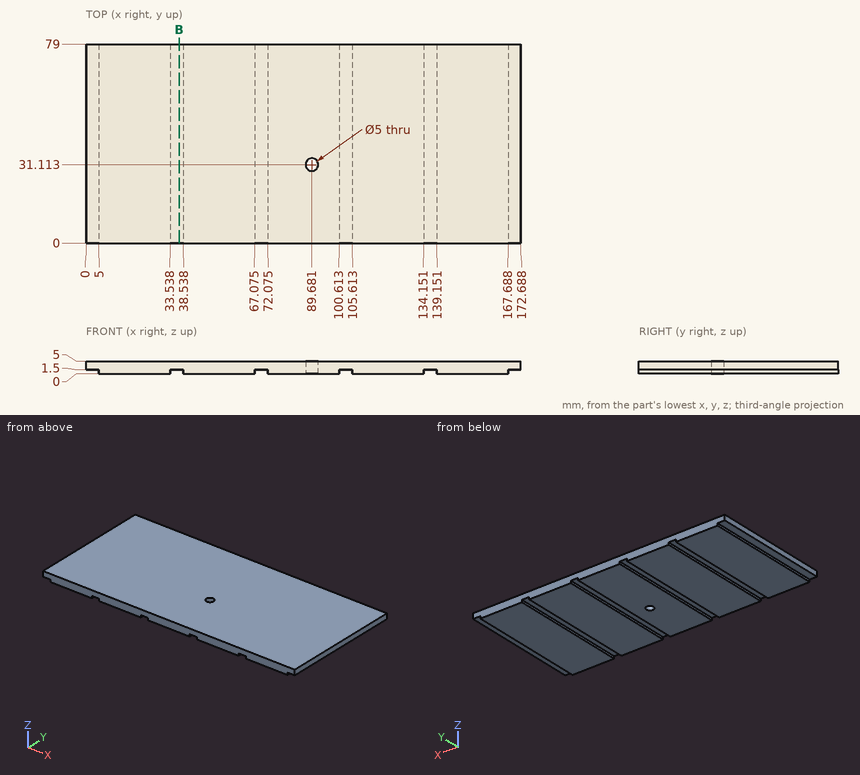
Can you work these out from the drawing? Everything is in mm from the part's minimum corner. Give positions to 0.01 mm unless a question says otherwise; leave off trailing zeros. Order: outer loops, then holes, each group sorted by start corner. A loop starts at its lowest first (then second) coordinate and runs counter-clockwise, first axis right, second up. Notation, with made-up numbers: M 38,65.25 L 72,65.25 A26 cw 72,91.25 Z; hole C 45,37.5 d2. An arc over 180 degrees is marked long. Use a Markdown table: item, result. Add a question column.
1. Suppose I cut it at B-B (x = 37). List the corners of the cut face in (y, z) for me.
2. I need wall thicknesses on probe 1 along X at (y, z) = (31.5, 4.45); probe 2 along Z at (x, y) = (37, 34); probe 3 along X at (y, z) = (29.5, 3.15). Which ranges of each line are inside material? Lowest first, please. Write a range as from..to.
3. For pin 1 Ø2.5 at (x, y) = (102.5, 34) entering from -Z; pin 2 Ø0.8 at (y, z) = (27.5, 1) entering from +X; pin 3 Ø0.8 at (y, z) = (47, 0.5) entering from -X, each with a flat end and sliding along its axis, tell me the tip position at first contact or that it passes through.
Results list:
| question | item | result |
|---|---|---|
| 1 | outline | M 0,1.5 L 79,1.5 L 79,5 L 0,5 Z |
| 2 | probe 1 | x = 0..87.21, 92.15..172.69 |
| 2 | probe 2 | z = 1.5..5 |
| 2 | probe 3 | x = 0..87.77, 91.59..172.69 |
| 3 | pin 1 | stops at z = 1.5 |
| 3 | pin 2 | stops at x = 167.69 |
| 3 | pin 3 | stops at x = 5 |
